Here's how the part is built. I have some questions about the finished solid (model axes, mm). Face numbers are marked on the shaded views. A direction names the side the tool comes from. Give positions to 0.01 mm unless a question says otherwise; leave off trailing zeros. Write each loop counter-clockwise with the first axis right and the second up, starting at its lowest first coordinate (ties: lowest second). Pieces come first, ordered by that corner, then holes. Notation, with made-up numbers: (-5.5, 76.5) -> (35.5, 76.5) arc R11 ccw to (35.5, 80.5) -> close; hole circle Ø6 at (53.25, 11). An arc over 180 degrees is marked (long way). Return JSON: item names as keys, results as strings.
from build123d import *
from build123d import SkipClean  # not in build123d's __all__

# Parameters (mm, degrees)
F0_W     = 30
F0_H     = 15
F1_DEPTH = 20
F3_DEPTH = 15.001
F2_R     = 5
F4_DEPTH = 15.001
F5_DEPTH = 5
F6_W     = 10
F6_H     = 5
F7_DEPTH = 30.001
F9_DEPTH = 15.001


with BuildPart() as f1:
    # F0 (on Top) → F1 (new body)
    with BuildSketch(Plane.XY):
        with Locations((15, 12.5)):
            Rectangle(F0_W, F0_H)
    extrude(amount=F1_DEPTH)

    # F2 (on face) → F3 (cut, through all)
    with BuildSketch(Plane.XZ.offset(-5)):
        Polygon((30, 14.8924803361), (30, 20), (25, 20), align=None)
        Polygon((30, 0), (30, 5), (25, 0), align=None)
    extrude(amount=-F3_DEPTH, mode=Mode.SUBTRACT)

    # F2 (on face) → F4 (cut, through all)
    with BuildSketch(Plane.XZ.offset(-5)):
        with Locations((10, 10)):
            Circle(F2_R)
    extrude(amount=-F4_DEPTH, mode=Mode.SUBTRACT)

    # F2 (on face) → F5 (join)
    with BuildSketch(Plane.XZ.offset(-5)):
        with BuildLine():
            ThreePointArc((20, 10), (17.0710678119, 17.0710678119), (10, 20))
            ThreePointArc((10, 20), (2.9289321881, 17.0710678119), (0, 10))
            ThreePointArc((0, 10), (2.9289321881, 2.9289321881), (10, 0))
            ThreePointArc((10, 0), (17.0710678119, 2.9289321881), (20, 10))
        make_face()
        with Locations((10, 10)):
            Circle(F2_R, mode=Mode.SUBTRACT)
    extrude(amount=F5_DEPTH)

    # F6 (on face) → F7 (cut, through all)
    with BuildSketch(Plane.YZ.offset(30)):
        with Locations((5, 9.8924803361)):
            Rectangle(F6_W, F6_H)
    extrude(amount=-F7_DEPTH, mode=Mode.SUBTRACT)

    # F8 (on face) → F9 (cut, through all)
    with BuildSketch(Plane.XZ.offset(-5)):
        with BuildLine():
            Line((0, 20), (0, 10))
            ThreePointArc((0, 10), (2.9289321881, 17.0710678119), (10, 20))
            Line((10, 20), (0, 20))
        make_face()
        with BuildLine():
            Line((0, 10), (0, 0))
            Line((0, 0), (10, 0))
            ThreePointArc((10, 0), (2.9289321881, 2.9289321881), (0, 10))
        make_face()
    with SkipClean():  # cleaning this boolean's faces spoils the solid; the shape is the same uncleaned
        extrude(amount=-F9_DEPTH, mode=Mode.SUBTRACT)


solid = f1.part
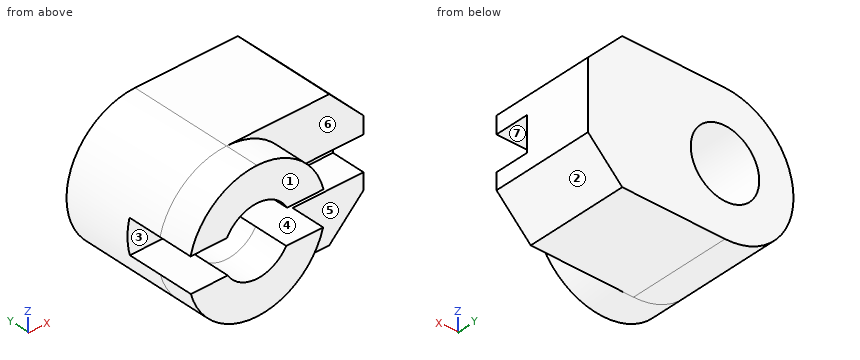
1. Suppose I cut it at D-D, the plane y = 11.25. List the corners of the cut face in (x, z) for me.
Taken from the geometry:
{"outline": "(10, 0) -> (25, 0) -> (30, 5) -> (30, 14.89) -> (25, 20) -> (10, 20) arc R10 ccw to start; hole circle Ø10 at (10, 10)"}
2. Suppose I cut it at C-C, the plane x = 12. List the corners of the cut face in (y, z) for me, and give its area (3 significant figures).
Taken from the geometry:
{"outline": "(0, 0.2) -> (5, 0.2) -> (5, 0) -> (20, 0) -> (20, 5.42) -> (0, 5.42) -> close; (0, 14.58) -> (20, 14.58) -> (20, 20) -> (5, 20) -> (5, 19.8) -> (0, 19.8) -> close", "area": "215 mm²"}
3. Suppose I cut it at B-B, the plane z = 10. List the corners of the cut face in (x, y) for me, and give its area (3 significant figures).
Taken from the geometry:
{"outline": "(0, 10) -> (5, 10) -> (5, 20) -> (0, 20) -> close; (15, 10) -> (30, 10) -> (30, 20) -> (15, 20) -> close", "area": "200 mm²"}
4. If I drill on line 1 (Z direction, x = 22, y = 7); line 2 (Z direction, x = 10, y = 12.25); line 3 (X direction, y = 19.25, z = 10), over which ranges is the centre line in solid material (lowest first)? Write a range as [from, to].
Taken from the geometry:
{"line 1": "z = [0, 7.39], [12.39, 20]", "line 2": "z = [0, 5], [15, 20]", "line 3": "x = [0, 5], [15, 30]"}
5. If we mould it in two halves opening along Z, with no side actions, what happens to the marked faces 1, 2, 3 and 4? For each: released by +Z, released by -Z, zero draft, split by the parting line, or undercut.
Taken from the geometry:
{"face 1": "zero draft", "face 2": "released by -Z", "face 3": "undercut", "face 4": "undercut"}
6. Suppose I cut it at A-A, the plane y = 7. List the corners of the cut face in (x, z) for me.
Taken from the geometry:
{"outline": "(0.29, 12.39) -> (5.61, 12.39) arc R5 cw to (14.39, 12.39) -> (30, 12.39) -> (30, 14.89) -> (25, 20) -> (10, 20) arc R10 ccw to start; (0.35, 7.39) arc R10 ccw to (10, 0) -> (25, 0) -> (30, 5) -> (30, 7.39) -> (14.27, 7.39) arc R5 cw to (5.73, 7.39) -> close"}
7. For pin 1 Ø1.5 at (x, z) = (13, 9.5) entering from +Y; pin 2 Ø2.5 at (x, z) = (2, 11) entering from -Y; pin 3 Ø6 at (x, z) = (26.5, 11.5) entering from -Y; pin 4 Ø6 at (y, z) = (9, 5.5) entering from -X, each with a flat end and sliding along its axis, tell me the tip position at first contact or that it passes through.
Taken from the geometry:
{"pin 1": "passes through", "pin 2": "stops at y = 10", "pin 3": "stops at y = 5", "pin 4": "stops at x = 0.14"}
8. Which directions (+Z, -Z, +X, -X, +Y, -Y) give clear straight access to the entire face, cutting with the end or side of a thin tool? Please do the marked faces 5, 6 and 7.
Taken from the geometry:
{"face 5": "-Z, +X, -Y", "face 6": "+Z, +X, -Y", "face 7": "+X, -X, -Y"}
